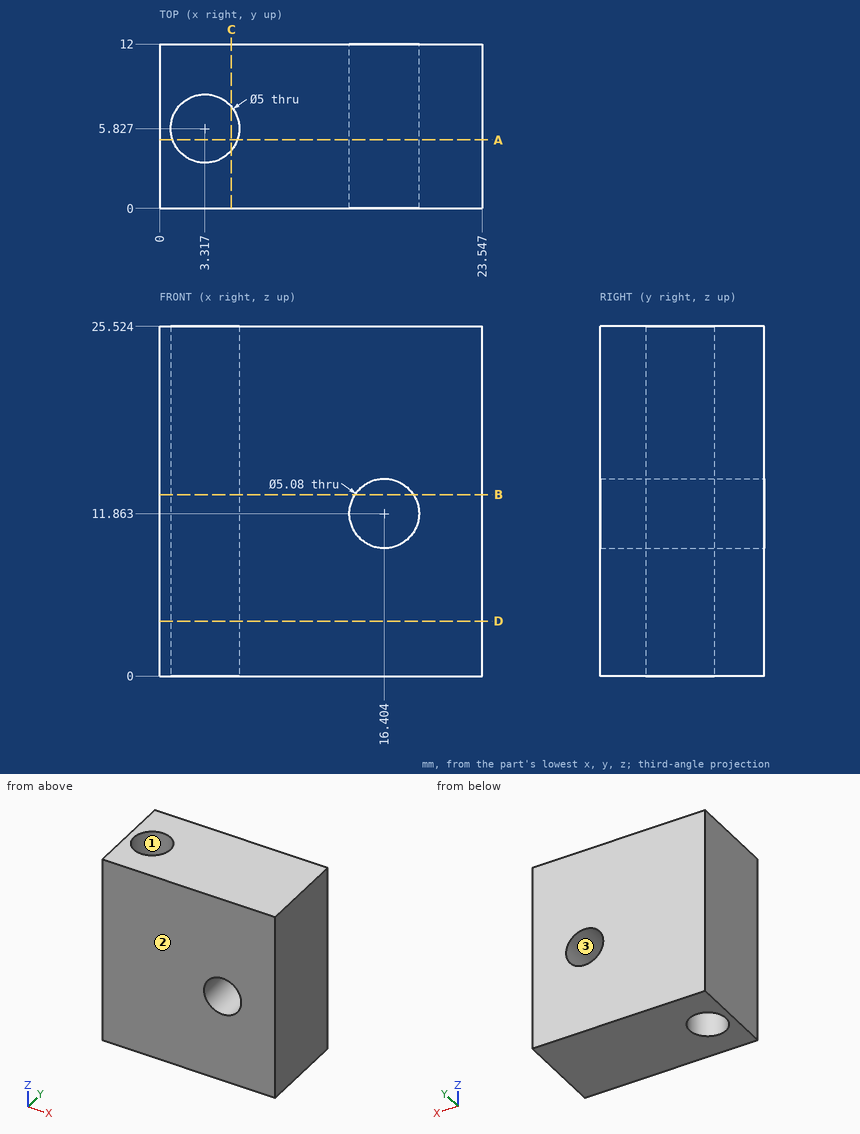
Verification items for this drawing (mm, ordinates from the low corner). Coordinates: 2 decimals unless noted, no trailing zeros. Loops run counter-clockwise (first coordinate to the right, second up) from the corner with the lowest first, then second, coordinate; pieces in that order, holes last. Notation, with made-up numbers: (-30, 76) -> (-10, 76) arc R26 cw to (-10, 107) -> close; hole circle Ø7 at (56.25, 42.25). An arc over 180 degrees is marked (long way). Put each result on its own line as item: value.
1. Section check A-A, the plane y = 5. Record the boundary of the cut face in (x, z) (1 decimal).
Result set:
outline: (0, 0) -> (1, 0) -> (1, 25.5) -> (0, 25.5) -> close; (5.7, 0) -> (23.5, 0) -> (23.5, 25.5) -> (5.7, 25.5) -> close; hole circle Ø5.1 at (16.4, 11.9)
2. Section check C-C, the plane x = 5.25. Record the boundary of the cut face in (y, z) (1 decimal), then the cut area to 3 significant figures.
Result set:
outline: (0, 0) -> (4.2, 0) -> (4.2, 25.5) -> (0, 25.5) -> close; (7.4, 0) -> (12, 0) -> (12, 25.5) -> (7.4, 25.5) -> close
area: 225 mm^2
3. Thickness scan on line 1 (Z direction, x = 16.25, y = 5.25) (1 decimal); line 2 (X direction, y = 6.5, z = 13.5) (1 decimal); line 3 (Y direction, x = 5.5, z = 14) (1 decimal). Record the ranges inside material, lowest first.
Result set:
line 1: z = 0 to 9.3, 14.4 to 25.5
line 2: x = 0 to 0.9, 5.7 to 14.5, 18.3 to 23.5
line 3: y = 0 to 4.6, 7 to 12
4. Section check D-D, the plane z = 4. Record the boundary of the cut face in (x, y).
Result set:
outline: (0, 0) -> (23.55, 0) -> (23.55, 12) -> (0, 12) -> close; hole circle Ø5 at (3.32, 5.83)
5. Section check B-B, the plane z = 13.25. Record the boundary of the cut face in (x, y).
Result set:
outline: (0, 0) -> (14.28, 0) -> (14.28, 12) -> (0, 12) -> close; (18.53, 0) -> (23.55, 0) -> (23.55, 12) -> (18.53, 12) -> close; hole circle Ø5 at (3.32, 5.83)
6. Mould release check, pull along Y, two halves, no side actions. Record for the marked faces 1, 2 and 3: pulls with the +Y half, pulls with the -Y half, needs draft (parallel to the pull), parting line crosses it, or undercut.
Result set:
face 1: undercut
face 2: pulls with the -Y half
face 3: needs draft
